from build123d import *

# Parameters (mm, degrees)
SKETCH1_W                        = 76.2
SKETCH1_H                        = 50.8
BOSS_EXTRUDE1_DEPTH              = 4.7625
F_17_32_0_53125_DIAMETER_HOLE1_D = 13.49375
F_1_8_0_125_DIAMETER_HOLE1_D     = 3.175
H_0_266_DIAMETER_HOLE1_D         = 6.7564


with BuildPart() as part:
    # Sketch1 → Boss-Extrude1 (new body)
    with BuildSketch(Plane.XY):
        Rectangle(SKETCH1_W, SKETCH1_H)
    extrude(amount=BOSS_EXTRUDE1_DEPTH)

    # 17/32 (0.53125) Diameter Hole1 (through all)
    with Locations(Plane.XY.offset(4.7625)):
        with Locations((-12.7, -6.35)):
            Hole(F_17_32_0_53125_DIAMETER_HOLE1_D / 2)

    # 1/8 (0.125) Diameter Hole1 (through all)
    with Locations(Plane.XY.offset(4.7625)):
        with Locations((-20.3454, 14.22428539), (-28.2702, 0.6604), (-20.6248, -12.74216218), (2.8702, 0.6604)):
            Hole(F_1_8_0_125_DIAMETER_HOLE1_D / 2)

    # H (0.266) Diameter Hole1 (through all)
    with Locations(Plane.XY.offset(4.7625)):
        with Locations((27.94, 12.7), (27.94, -12.7)):
            Hole(H_0_266_DIAMETER_HOLE1_D / 2)


solid = part.part
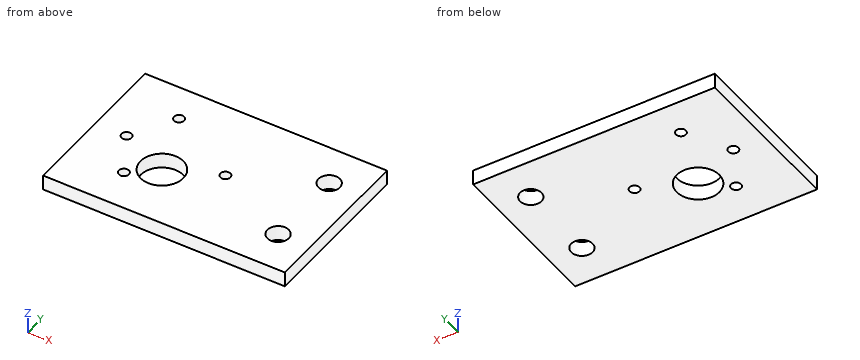
For this review, take the finished solid that the model builds, in its own axes (mm). Round coordinates to 2 decimals unless told otherwise and drop trailing zeros. Order: outer loops, then holes, each group sorted by start corner. A loop starts at its lowest first (then second) coordinate and runs counter-clockwise, first axis right, second up. Notation, with made-up numbers: M -29,22.5 L 20,22.5 A16 cw 20,31.5 Z; hole C -17.75,-9.5 d8. An arc over 180 degrees is marked long. Use a Markdown table: item, result. Add a question column.
Item 1: Add section A-A, the plane x = -12.7. Give the boundary of the cut face in (y, z), then the cut area to 3 significant figures.
Item 2: To check wall thickness, follow line 1 along Y through (x, z) = (27.94, 2.35); line 2 along X through (y, z) = (12.5, 3.5); line 3 along X through (y, z) = (-10, 1.2). State the ranges of each line that lie inside material, in increasing order.
Item 3: Add section C-C, the plane y = -6.35. Give the boundary of the cut face in (x, z), then the cut area to 3 significant figures.
Item 4: Add section B-B, the plane x = 27.94. Give the boundary of the cut face in (y, z), then the cut area to 3 significant figures.
Item 5: Add section D-D, the plane z = 1.85. State how many separate pieces and enclosed holes the cut face has, then the cut area to 3 significant figures.
Geometry results:
| question | item | result |
|---|---|---|
| 1 | outline | M -25.4,0 L -13.1,0 L -13.1,4.76 L -25.4,4.76 Z; M 0.4,0 L 25.4,0 L 25.4,4.76 L 0.4,4.76 Z |
| 1 | area | 178 mm² |
| 2 | line 1 | y = -25.4 to -16.08, -9.32 to 9.32, 16.08 to 25.4 |
| 2 | line 2 | x = -38.1 to 24.57, 31.31 to 38.1 |
| 2 | line 3 | x = -38.1 to -18.37, -7.03 to 25.91, 29.97 to 38.1 |
| 3 | outline | M -38.1,0 L -19.45,0 L -19.45,4.76 L -38.1,4.76 Z; M -5.95,0 L 38.1,0 L 38.1,4.76 L -5.95,4.76 Z |
| 3 | area | 299 mm² |
| 4 | outline | M -25.4,0 L -16.08,0 L -16.08,4.76 L -25.4,4.76 Z; M -9.32,0 L 9.32,0 L 9.32,4.76 L -9.32,4.76 Z; M 16.08,0 L 25.4,0 L 25.4,4.76 L 16.08,4.76 Z |
| 4 | area | 178 mm² |
| 5 | separate pieces | 1 |
| 5 | enclosed holes | 7 |
| 5 | area | 3,620 mm² |
